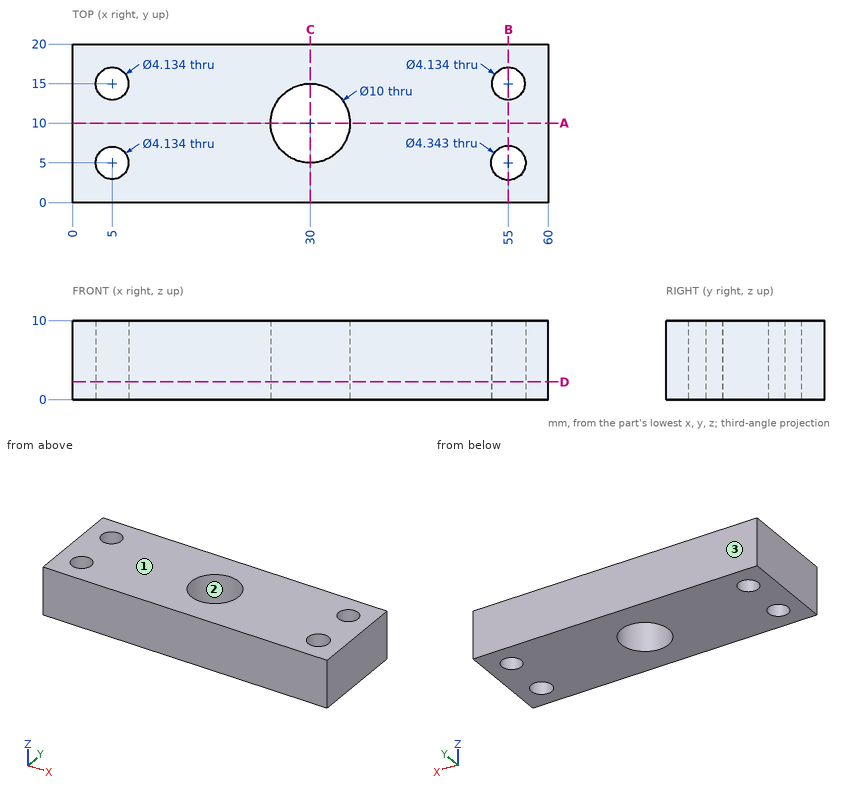
Job drawing, mm, ordinate dimensions from the low corner. One solid piece. Round coordinates to 2 decimals unless told otherwise and drop trailing zeros. Loops run counter-clockwise (first coordinate to the right, second up) from the corner with the lowest first, then second, coordinate; pieces in that order, holes last. Notation, with made-up numbers: (-37.5, 47) -> (7.5, 47) arc R22 cw to (7.5, 59) -> close; hole circle Ø2 at (25, -33.5). An arc over 180 degrees is marked (long way). One line per item, written item: value. Start each with the question number.
Q1. Probe line 1 along Y through (x, z) = (55, 2.5); line 2 along Y through (x, z) = (5, 4.25); line 3 along X through (y, z) = (10.25, 4.25). List the from-to ranges inside material, lowest first.
Q2. Cut at B-B on x = 55. List the corners of the cut face in (y, z).
Q3. Cut at C-C on x = 30. List the corners of the cut face in (y, z), plus the area to 3 significant figures.
Q4. Two-plate mould, pull along Y, no slides. Class the marked faces 1, 2 and 3: released by +Y, released by -Y, zero draft, split by the parting line, or undercut.
Q5. Cut at A-A on y = 10. List the corners of the cut face in (x, z).
Q6. Drop a flat-ended pin along its axis: pin 1 Ø9 at (x, y) = (30, 10) entering from +Z. Give the stop position or say it passes through.
Q7. Cut at D-D on z = 2.25. List the corners of the cut face in (x, y), plus the area to 3 significant figures.
Computed:
1. line 1: 0 to 2.83, 7.17 to 12.93, 17.07 to 20
1. line 2: 0 to 2.93, 7.07 to 12.93, 17.07 to 20
1. line 3: 0 to 25.01, 34.99 to 60
2. outline: (0, 0) -> (2.83, 0) -> (2.83, 10) -> (0, 10) -> close; (7.17, 0) -> (12.93, 0) -> (12.93, 10) -> (7.17, 10) -> close; (17.07, 0) -> (20, 0) -> (20, 10) -> (17.07, 10) -> close
3. outline: (0, 0) -> (5, 0) -> (5, 10) -> (0, 10) -> close; (15, 0) -> (20, 0) -> (20, 10) -> (15, 10) -> close
3. area: 100 mm²
4. face 1: zero draft
4. face 2: undercut
4. face 3: released by +Y
5. outline: (0, 0) -> (25, 0) -> (25, 10) -> (0, 10) -> close; (35, 0) -> (60, 0) -> (60, 10) -> (35, 10) -> close
6. pin 1: through
7. outline: (0, 0) -> (60, 0) -> (60, 20) -> (0, 20) -> close; hole circle Ø4.13 at (5, 5); hole circle Ø4.13 at (5, 15); hole circle Ø10 at (30, 10); hole circle Ø4.34 at (55, 5); hole circle Ø4.13 at (55, 15)
7. area: 1,070 mm²
